Source: CAD feature listing. Evaluate the final solid. Frame: model axes, mm. Face numbers are marked on the shaded views. A direction names the side the tool comes from. Coordinates: 2 decimals unless noted, no trailing zeros. Order: outer loops, then holes, each group sorted by start corner. A loop starts at its lowest first (then second) coordinate and runs counter-clockwise, first axis right, second up.
Item 1: Section C-C on y = -37.5. Return the cut outline in (x, z), then the cut area to 3 significant figures.
Item 2: Reachability of the marked faces 1 and 2 from +Z, -Z, +X, -X, +Y, -Y: full face, straight path, thin tool, end or side. Return the list, or none.
Item 3: Section A-A on x = 0. Return the cut outline in (y, z), then the cut area to 3 significant figures.
Item 4: Section B-B on z = 0. Return the cut outline in (x, y), then the cut area to 3 significant figures.
Item 5: Contact query for flat-ended pins moving along their axis: P1, Ø1, axis at y = -48, z = 1, coming from the +X side; P2, Ø1, axis at y = -40, z = 2.5, coming from the -X side. Output: stop coordinate, or through.
Item 6: Section D-D on y = -101. Return the cut outline in (x, z).
Item 7: Ray query, line 1 (Z direction, x = -0.5, y = -101); line 2 (Y direction, x = -1.25, z = 0); line 3 (Z direction, x = -4.5, y = -71). Return the intervals inside material, ascending.
from build123d import *

# Parameters (mm, degrees)
F0_R     = 6
F1_DEPTH = 106
F2_SIZE  = 0.5
F3_W     = 20
F3_H     = 5
F4_DEPTH = 10
F5_R     = 1.5
F6_DEPTH = 12.5


with BuildPart() as f1:
    # F0 (on Front) → F1 (new body)
    with BuildSketch(Plane.XZ):
        Circle(F0_R)
    extrude(amount=F1_DEPTH)

    # F2
    f2_edges = [f1.edges().sort_by_distance(p)[0] for p in [
        (-6, -106, 0),
        (-6, 0, 0),
    ]]
    chamfer(f2_edges, length=F2_SIZE)

    # F3 (on Front) → F4 (cut)
    with BuildSketch(Plane.XZ):
        with Locations((0, 7)):
            Rectangle(F3_W, F3_H)
    extrude(amount=F4_DEPTH, mode=Mode.SUBTRACT)

    # F5 (on Right) → F6 (cut, symmetric)
    with BuildSketch(Plane.YZ):
        with Locations((-101, 0)):
            Circle(F5_R)
    extrude(amount=F6_DEPTH, both=True, mode=Mode.SUBTRACT)


solid = f1.part
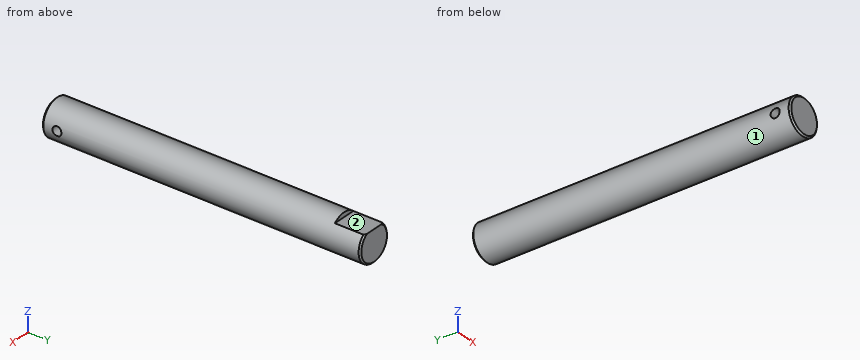
Answer list:
1. outline: circle Ø12 at (0, 0)
1. area: 113 mm2
2. face 1: +Y, -Y
2. face 2: +Z, +X, -X, +Y
3. outline: (-106, -5.5) - (-105.5, -6) - (-0.5, -6) - (0, -5.5) - (0, 4.5) - (-10, 4.5) - (-10, 6) - (-105.5, 6) - (-106, 5.5) - close; hole circle Ø3 at (-101, 0)
3. area: 1,250 mm2
4. outline: (-6, -105.5) - (-5.5, -106) - (5.5, -106) - (6, -105.5) - (6, -102.5) - (-6, -102.5) - close; (-6, -99.5) - (6, -99.5) - (6, -0.5) - (5.5, 0) - (-5.5, 0) - (-6, -0.5) - close
4. area: 1,240 mm2
5. P1: stops at x = 5.98
5. P2: stops at x = -5.66
6. outline: (-5.81, -1.5) arc R6 ccw to (5.81, -1.5) - close; (-5.81, 1.5) - (5.81, 1.5) arc R6 ccw to start
7. line 1: z = -5.98 to -1.5, 1.5 to 5.98
7. line 2: y = -106 to -102.5, -99.5 to 0
7. line 3: z = -3.97 to 3.97
